Autodesk Inventor part; units mm, degrees
ref_plane "YZ Plane" through (0, 0, 0) normal (1, 0, 0) x (0, 1, 0)
ref_plane "XZ Plane" through (0, 0, 0) normal (0, 1, 0) x (-1, 0, 0)
ref_plane "XY Plane" through (0, 0, 0) normal (0, 0, 1) x (1, 0, 0)
sketch "Sketch1" plane through (0, 0, 0) normal (0, 0, 1) x (1, 0, 0)
  line L0 (0, 0) -> (25.4, 0)
  line L1 (25.4, 0) -> (25.4, 25.4)
  line L2 (25.4, 25.4) -> (0, 25.4)
  line L3 (0, 25.4) -> (0, 0)
  line L4 (3.175, 22.225) -> (22.225, 22.225)
  line L5 (22.225, 22.225) -> (22.225, 3.175)
  line L6 (22.225, 3.175) -> (3.175, 3.175)
  line L7 (3.175, 3.175) -> (3.175, 22.225)
  dimension "d0" = 25.4
  dimension "d1" = 25.4
  dimension "d2" = 3.175
extrude "Extrusion1" add sketch "Sketch1" along normal blind 76.2
sketch "Sketch2" plane through (0, 25.4, 0) normal (0, 1, 0) x (1, 0, 0)
  line L0 (3.175, 0) -> (22.225, 0) construction
  line L1 (12.7, 0) -> (12.7, -12.7) construction
  line L2 (0, -76.2) -> (25.4, -76.2) construction
  line L3 (12.7, -76.2) -> (12.7, -63.5) construction
  circle A0 centre (12.7, -63.5) radius 2.5797
  circle A1 centre (12.7, -12.7) radius 2.5797
  point P0 (0, 0)
  dimension "d5" = 12.7
  dimension "d6" = 12.7
  dimension "d7" = 5.1594
extrude "Extrusion2" cut sketch "Sketch2" against normal blind 76.2
sketch "Sketch3" plane through (25.4, 0, 0) normal (1, 0, 0) x (0, 0, -1)
  line L0 (0, 22.225) -> (0, 3.175)
  line L1 (0, 12.7) -> (-12.7, 12.7) construction
  line L2 (-76.2, 3.175) -> (-76.2, 22.225)
  line L3 (-76.2, 12.7) -> (-63.5, 12.7) construction
  circle A0 centre (-63.5, 12.7) radius 2.5797
  circle A1 centre (-12.7, 12.7) radius 2.5797
  point P0 (0, 0)
  dimension "d10" = 12.7
  dimension "d11" = 12.7
  dimension "d12" = 5.1594
extrude "Extrusion3" cut sketch "Sketch3" against normal blind 76.2
properties part number "1x1 3in"
The model under review builds one solid part; all positions refer to its coordinate system, in mm. A direction names the side the tool comes from. Give positions to 0.01 mm unless a question says otherwise; leave off trailing zeros. Write each loop counter-clockwise with the first axis right and the second up, starting at its lowest first coordinate (ties: lowest second). Pieces come first, ordered by that corner, then holes. Notation, with made-up numbers: M -11,39 L -4,39 A38 cw -4,78 Z; hole C -28,78.5 d5. An arc over 180 degrees is marked long. Write item = value, one per line. Start each with the question number.
Q1. We need section B-B (y = 19). State the section outline as (x, z) points (3 decimals).
Q2. We need section A-A (x = 12.7). State the section outline as (y, z) points (3 decimals).
Q3. We need section C-C (z = 17). State the section outline as (x, y) points (3 decimals), plus the area to 3 significant figures.
Q4. For line 1 (X direction, y = 17.5, z = 17) (3 decimals); line 2 (X direction, y = 23.15, z = 12.7), list the stretches that pass through material, from the lowest coordinate up.
Q5. Mouldability with a two-part tool opening along Z and no side actions: class faces 1 (the face through (24, 13, 0)), 2 (the face through (14.087, 1.61, 10.525)), 3 (the face through (13, 0, 38)) as released by +Z, released by -Z, zero draft, split by the parting line, or undercut.
Q6. Machinability: for faces 4 (the face through (3.175, 13, 38)), 5 (the face through (24, 13, 76.2)), which of the approach directions +Z, -Z, +X, -X, +Y, -Y give a long, thin tool a straight path to every point of the face, cutting with its end or side? Answer none if there is none.
Result set:
q1.outline = M 0,0 L 3.175,0 L 3.175,76.2 L 0,76.2 Z; M 22.225,0 L 25.4,0 L 25.4,76.2 L 22.225,76.2 Z
q2.outline = M 0,0 L 3.175,0 L 3.175,10.12 L 0,10.12 Z; M 0,15.28 L 3.175,15.28 L 3.175,60.92 L 0,60.92 Z; M 0,66.08 L 3.175,66.08 L 3.175,76.2 L 0,76.2 Z; M 22.225,0 L 25.4,0 L 25.4,10.12 L 22.225,10.12 Z; M 22.225,15.28 L 25.4,15.28 L 25.4,60.92 L 22.225,60.92 Z; M 22.225,66.08 L 25.4,66.08 L 25.4,76.2 L 22.225,76.2 Z
q3.outline = M 0,0 L 25.4,0 L 25.4,25.4 L 0,25.4 Z; hole M 3.175,3.175 L 22.225,3.175 L 22.225,22.225 L 3.175,22.225 Z
q3.area = 282 mm2
q4.line_1 = 0 to 3.175, 22.225 to 25.4
q4.line_2 = 0 to 10.12, 15.28 to 25.4
q5.face_1 = released by -Z
q5.face_2 = undercut
q5.face_3 = zero draft
q6.face_4 = +Z, -Z
q6.face_5 = +Z, +X, -X, +Y, -Y
